Read the model definition and answer for the solid it produces. Units are mm, in the model's axes. Face numbers are marked on the shaded views. A direction names the side the tool comes from. Give positions to 0.01 mm unless a question says otherwise; leave off trailing zeros. Write each loop counter-clockwise with the first axis right and the second up, starting at its lowest first coordinate (ties: lowest second). Pieces come first, ordered by that corner, then holes. Notation, with made-up numbers: M 17,83 L 50,83 A28 ccw 50,101 Z; hole C -16,-22 d6. An arc over 180 degrees is marked long. Put each result on its own line as item: value.
Autodesk Inventor part; units mm, degrees
ref_plane "YZ Plane" through (0, 0, 0) normal (1, 0, 0) x (0, 1, 0)
ref_plane "XZ Plane" through (0, 0, 0) normal (0, 1, 0) x (-1, 0, 0)
ref_plane "XY Plane" through (0, 0, 0) normal (0, 0, 1) x (1, 0, 0)
sketch "Sketch1" plane through (0, 0, 0) normal (0, 1, 0) x (-1, 0, 0)
  circle A0 centre (0, 0) radius 60
  dimension "d0" = 120
extrude "Extrusion1" add sketch "Sketch1" along normal blind 2.5
sketch "Sketch2" plane through (0, 0, 0) normal (0, 0, 1) x (1, 0, 0)
  line L0 (60, 2.5) -> (-60, 2.5)
  line L1 (-10, 17.5) -> (-4, 17.5)
  line L2 (10, 17.5) -> (10, 2.5)
  line L3 (10, 2.5) -> (-10, 2.5)
  line L4 (-10, 2.5) -> (-10, 17.5)
  circle A0 centre (0, 17.5) radius 10
  circle A1 centre (0, 17.5) radius 4
  line L5 (4, 17.5) -> (10, 17.5)
  line L6 (-4, 17.5) -> (4, 17.5)
  point P0 (0, 0)
  point P1 (0, 2.5)
  dimension "d3" = 20
  dimension "d4" = 15
  dimension "d5" = 8
extrude "Extrusion2" add sketch "Sketch2" along normal mid plane 18 contours L0 L4 A0 L2 | L5 A1 L1 A0 | A0 L1 A1 L5
sketch "Sketch4" plane through (10, 2.5, 9) normal (1, 0, 0) x (0, 0, -1)
  line L0 (18, 15) -> (0, 15)
  line L1 (18, 15) -> (18, 15)
  line L2 (0, 15) -> (18, 15)
  line L3 (0, 15) -> (0, 15)
  line L4 (18, 15) -> (0, 15)
  line L5 (0, 0) -> (0, 15)
  line L6 (18, 0) -> (0, 0)
  line L7 (18, 15) -> (18, 0)
  line L8 (5, 25) -> (13, 25)
  line L9 (13, 25) -> (13, 0)
  line L10 (13, 0) -> (5, 0)
  line L11 (5, 0) -> (5, 25)
  line L12 (69, 0) -> (-51, 0)
  point P0 (9, -2.5)
  point P1 (9, 0)
  dimension "d8" = 8
  dimension "d9" = 25
extrude "Extrusion3" cut sketch "Sketch4" against normal blind 20 contours L9 L6 L11 L0 | L0 L11 L8 L9
sketch "Sketch5" plane through (0, 2.5, 0) normal (0, 1, 0) x (1, 0, 0)
  line L0 (10, -4) -> (10, -9)
  line L1 (10, -9) -> (-10, -9)
  line L2 (-10, -9) -> (-10, -4)
  line L3 (10, -4) -> (-10, -4)
  line L4 (10, 4) -> (-10, 4)
  line L5 (-10, 4) -> (-10, 9)
  line L6 (-10, 9) -> (10, 9)
  line L7 (10, 9) -> (10, 4)
  circle A0 centre (0, 0) radius 60
  line L8 (1, 3) -> (-1, 3)
  line L9 (-1, 3) -> (-1, -3)
  line L10 (-1, -3) -> (1, -3)
  line L11 (1, -3) -> (1, 3)
  line L12 (-1, -3) -> (1, 3) construction
  line L13 (-1, 3) -> (1, -3) construction
  line L14 (0, 0) -> (50, 0) construction
  line L15 (0, 0) -> (50, 0) construction
  line L16 (0, 0) -> (35.3553, 35.3553) construction
  line L17 (0, 0) -> (50, 0) construction
  line L18 (0, 0) -> (0, 50) construction
  line L19 (0, 0) -> (50, 0) construction
  line L20 (0, 0) -> (-35.3553, 35.3553) construction
  line L21 (0, 0) -> (50, 0) construction
  line L22 (0, 0) -> (-50, 0) construction
  line L23 (0, 0) -> (50, 0) construction
  line L24 (0, 0) -> (-35.3553, -35.3553) construction
  line L25 (0, 0) -> (50, 0) construction
  line L26 (0, 0) -> (0, -50) construction
  line L27 (0, 0) -> (50, 0) construction
  line L28 (0, 0) -> (35.3553, -35.3553) construction
  line L29 (0, 0) -> (50, 0) construction
  circle A1 centre (0, -50) radius 2.1
  circle A2 centre (35.3553, -35.3553) radius 2.1
  circle A3 centre (50, 0) radius 2.1
  circle A4 centre (35.3553, 35.3553) radius 2.1
  circle A5 centre (0, 50) radius 2.1
  circle A6 centre (-35.3553, 35.3553) radius 2.1
  circle A7 centre (-50, 0) radius 2.1
  circle A8 centre (-35.3553, -35.3553) radius 2.1
  point P0 (0, 0)
  dimension "d13" = 120
  dimension "d17" = 6
  dimension "d18" = 2
  dimension "d19" = 50
  dimension "d20" = 0
  dimension "d21" = 50
  dimension "d22" = 45
  dimension "d23" = 50
  dimension "d24" = 90
  dimension "d25" = 50
  dimension "d26" = 135
  dimension "d27" = 50
  dimension "d28" = 180
  dimension "d29" = 50
  dimension "d30" = 135
  dimension "d31" = 50
  dimension "d32" = 90
  dimension "d33" = 50
  dimension "d34" = 45
  dimension "d35" = 4.2
  dimension "d36" = 4.2
  dimension "d37" = 4.2
  dimension "d38" = 4.2
  dimension "d39" = 4.2
  dimension "d40" = 4.2
  dimension "d41" = 4.2
  dimension "d42" = 4.2
extrude "Extrusion4" cut sketch "Sketch5" against normal blind 20 contours L11 L10 L9 L8 | A1 | A2 | A4 | A5 | A6 | A7 | A8
equation "\"d36\" = d35"
equation "\"d37\" = d36"
equation "\"d38\" = d37"
equation "\"d39\" = d38"
equation "\"d40\" = d39"
equation "\"d41\" = d40"
equation "\"d42\" = d41"
properties part number "Base top" material "ABS Plastic"
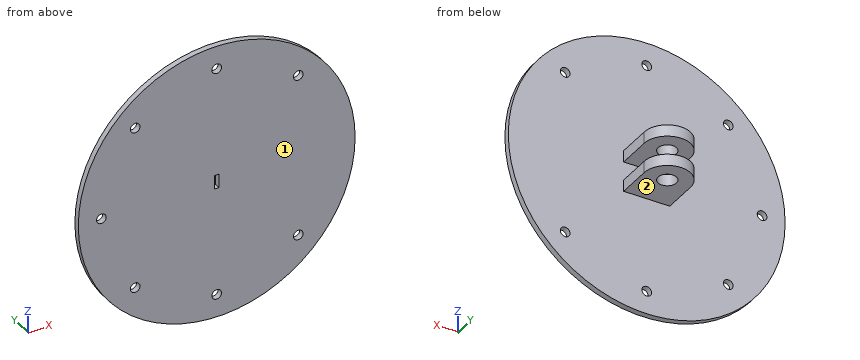
(1) Section C-C on z = -50 is taken. Determine the outline of the cut face in (x, y), and give its area (3 significant figures).
Result:
outline: M -33.17,0 L -2.1,0 L -2.1,2.5 L -33.17,2.5 Z; M 2.1,0 L 33.17,0 L 33.17,2.5 L 2.1,2.5 Z
area: 155 mm²
(2) Section D-D on x = -7.5 is taken. Determine the outline of the cut face in (y, z), and give its area (3 significant figures).
Result:
outline: M 0,-59.53 L 2.5,-59.53 L 2.5,-9 L 24.11,-9 L 24.11,-4 L 2.5,-4 L 2.5,4 L 24.11,4 L 24.11,9 L 2.5,9 L 2.5,59.53 L 0,59.53 Z
area: 514 mm²
(3) Straight lines are drawn through the part: line 1 along Z through (x, y) = (0, 1.6); line 2 along Z through (x, y) = (6.5, 9); line 3 along X through (y, z) = (17.5, -5.35). For each, find the intervals that lie inside material, in ascending order. Write a range as from..to.
Result:
line 1: z = -60..-52.1, -47.9..-3, 3..47.9, 52.1..60
line 2: z = -9..-4, 4..9
line 3: x = -10..-4, 4..10
(4) Section A-A on y = 23.5 is taken. Determine the outline of the cut face in (x, z), and give its area (3 significant figures).
Result:
outline: M -8,-9 L 8,-9 L 8,-4 L -8,-4 Z; M -8,4 L 8,4 L 8,9 L -8,9 Z
area: 160 mm²
(5) Section B-B on z = 0 is taken. Determine the outline of the cut face in (x, y).
Result:
outline: M -60,0 L -52.1,0 L -52.1,2.5 L -60,2.5 Z; M -47.9,0 L -1,0 L -1,2.5 L -47.9,2.5 Z; M 1,0 L 60,0 L 60,2.5 L 1,2.5 Z
(6) Which of the six approach directions +Z, -Z, +X, -X, +Y, -Y give full straight-line access (tool end or side, diameter ignored) to the marked faces 1 and 2?
Result:
face 1: +Z, -Z, +X, -X, -Y
face 2: -Z, +X, -X, +Y
(7) Given pin 1 Ø4 at (x, z) = (16, -6.5) entering from +Y; pin 2 Ø1.6 at (x, y) = (0, 1) entering from +Z; pin 3 Ø4 at (y, z) = (8, 9.5) entering from -X; pin 4 Ø3.5 at (x, z) = (35.36, -35.36) entering from +Y, each flat-ended and moving along its own axis, determine where each tip first touches the part or whether it passes through.
Result:
pin 1: stops at y = 2.5
pin 2: stops at z = 60
pin 3: stops at x = -10
pin 4: passes through
